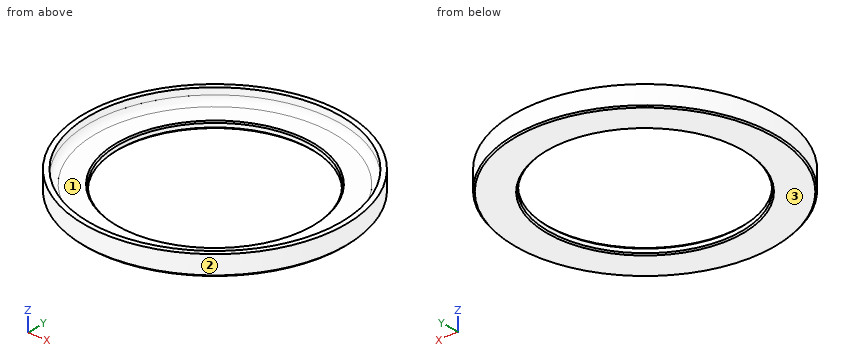
Autodesk Fusion 360 part; units mm, degrees
sketch "Sketch1" plane through (0, 0, 0) normal (0, 0, 1) x (1, 0, 0)
  circle A0 centre (0, 0) radius 14.6
  circle A1 centre (0, 0) radius 19
  circle A2 centre (0, 0) radius 19.75
  dimension "d1" = 29.2
  dimension "d2" = 38
  dimension "d3" = 39.5
extrude "Extrude3" add sketch "Sketch1" along normal blind 1 contours A1
extrude "Extrude4" add sketch "Sketch1" along normal blind 3 contours A2
fillet "Fillet1" radius 1 1 edges at (-17.7142, -6.8707, 1)
chamfer "Chamfer1" distance 0.2 angle 45 1 edges at (-18.4135, -7.1419, 0)
chamfer "Chamfer2" distance 0.2 angle 45 2 edges at (-13.612, 5.2796, 1) (-13.612, 5.2796, 0)
extrude "Extrude1" [suppressed]
extrude "Extrude2" [suppressed]
Verification items for the finished model (mm, model axes). Face numbers are marked on the shaded views. Coordinates: 2 decimals unless noted, no trailing zeros. Order: outer loops, then holes, each group sorted by start corner. A loop starts at its lowest first (then second) coordinate and runs counter-clockwise, first axis right, second up.
Item 1: Material ranges on L1, parallel to Y at x = 0, z = 0.5; L2, parallel to Y at x = 0, z = 2.65; L3, parallel to Z at x = -14.5, y = 6.5, recorded low to high.
Filled in:
L1: y = -19.75 to -14.6, 14.6 to 19.75
L2: y = -19.75 to -19, 19 to 19.75
L3: z = 0 to 1
Item 2: Section check C-C, the plane z = 2.45. Enter the section's corners in (x, y), then the cut area to 3 significant figures.
Filled in:
outline: circle Ø39.5 at (0, 0); hole circle Ø38 at (0, 0)
area: 91.3 mm2
Item 3: Depth check by flat-ended pin: pin 1 (5 mm diameter, centred on x = 14.5, y = 0.5, fed in from +Z); pin 2 (1 mm diameter, centred on x = 3.5, z = 1, fed in from -Y). Enter the tip coordinate at first touch or a pass-through.
Filled in:
pin 1: stops at z = 1
pin 2: stops at y = -19.52
Item 4: Release check for a two-part mould opening along Y. For the marked faces 1, 2 and 3 record: +Y half, -Y half, draft (parallel to the pull), parting line (faces both ways), or undercut.
Filled in:
face 1: undercut
face 2: parting line
face 3: draft
Item 5: Section check A-A, the plane x = 0. Enter the section's corners in (y, z), then the cut area to 3 significant figures.
Filled in:
outline: (-19.75, 0.2) - (-19.55, 0) - (-14.8, 0) - (-14.6, 0.2) - (-14.6, 0.8) - (-14.8, 1) - (-18, 1) arc R1 cw to (-19, 2) - (-19, 3) - (-19.75, 3) - close; (14.6, 0.2) - (14.8, 0) - (19.55, 0) - (19.75, 0.2) - (19.75, 3) - (19, 3) - (19, 2) arc R1 cw to (18, 1) - (14.8, 1) - (14.6, 0.8) - close
area: 13.6 mm2
